Verification items for the finished model (mm, model axes). A direction names the side the tool comes from. Give positions to 0.01 mm unless a question says otherwise; leave off trailing zeros. Loops run counter-clockwise (first coordinate to the right, second up) from the corner with the lowest first, then second, coordinate; pieces in that order, holes last. Notation, with made-up numbers: (-36.75, 0) -> (14.25, 0) arc R16 cw to (14.25, 8) -> close; hole circle Ø10 at (-36.5, 40.5). An arc over 180 degrees is marked (long way). Answer in a Markdown table with one row per item. Add a question column.
Q1. Section check C-C on z = 21.5. Enter the section's corners in (x, y) (3 decimals), and give its area (3 significant figures).
Q2. Gauge pin test, flat ends, axial feed: P1, Ø2, axis at y = -26.5, z = -1.5, coming from the +X side; P2, Ø3, axis at y = -48, z = 18, coming from the -X side; P3, Ø2, axis at x = -3, z = -0.5, coming from the +Y side; P4, Ø12, axis at x = -15, z = 11.5, coming from the +Y side. Record the tip position at first contact, or that the pin passes through.
Q3. Section check D-D on y = -11. Enter the section's corners in (x, z), and give its area (3 significant figures).
Q4. Section check A-A on x = 9.5. Enter the section's corners in (y, z), and give its area (3 significant figures).
Q5. Release check for a two-part mould opening along Y. For faces 4 (the face through (1, -54.61, 13)), 5 (the face through (19.05, -24, -1)), 6 (the face through (51.41, -1.61, 23.87)) record: pulls with the +Y half, pulls with the -Y half, needs draft (parallel to the pull), parting line crosses it, or undercut.
Q6. Material ranges on probe 1 along X at (y, z) = (-9.5, 5.75); probe 2 along X at (y, z) = (-56, 23); probe 3 along Z at (x, y) = (-15.5, -52), recorded low to high.
Q7. Set-up check for faces 1 (the face through (-48, -3.175, 12)), 2 (the face through (-1, -46, 0)), 3 (the face through (0, -41.91, -1)): record each of +Z, -Z, +X, -X, +Y, -Y from which the full face is reachable in a straight line by a thin tool's end or side.
Q8. Section check B-B on y = -4.5. Enter the section's corners in (x, z).
```python
from build123d import *

# Parameters (mm, degrees)
F1_DEPTH  = 25.4
F2_W      = 87.9329293966
F2_H      = 59.3619965534
F3_DEPTH  = 2.54
F4_W      = 8.89
F4_H      = 27.94
F5_DEPTH  = 3.175
F7_DEPTH  = 2.541
F8_R      = 5.08
F9_R      = 2.38125
F10_DEPTH = 3.176


# Not quite as in the source:
# - a feature names something its author has since deleted; it is built from what else it names


with BuildPart() as f1:
    # F0 (on Top) → F1 (new body)
    with BuildSketch(Plane.XY):
        Polygon((38.1, -54.61), (-38.1, -54.61), (-38.1, 0), (-43.9664646983, 0), (-43.9664646983, -59.3619965534), (43.9664646983, -59.3619965534), (43.9664646983, 0), (38.1, 0), align=None)
    extrude(amount=F1_DEPTH)

    # F2 (on face) → F3 (join)
    with BuildSketch(Plane(origin=(0, 0, 0), x_dir=(1, 0, 0), z_dir=(0, 0, -1))):
        with Locations((0, 29.6809982767)):
            Rectangle(F2_W, F2_H)
    extrude(amount=F3_DEPTH)

    # F4 (on face) → F5 (join)
    with BuildSketch(Plane(origin=(0, 0, 0), x_dir=(-1, 0, 0), z_dir=(0, 1, 0))):
        with Locations((-48.4114646983, 11.43)):
            Rectangle(F4_W, F4_H)
        with Locations((48.4114646983, 11.43)):
            Rectangle(F4_W, F4_H)
    extrude(amount=-F5_DEPTH)

    # F6 (on face) → F7 (cut, through all)
    with BuildSketch(Plane.XY):
        Polygon((0, -6.35), (-19.05, -6.35), (-19.05, -41.91), (0, -41.91), (19.05, -41.91), (19.05, -6.35), align=None)
    extrude(amount=-F7_DEPTH, mode=Mode.SUBTRACT)

    # F8
    f8_edges = [f1.edges().sort_by_distance(p)[0] for p in [
        (52.856465, -1.5875, 25.4),
        (-52.856465, -1.5875, 25.4),
        (-52.856465, -1.5875, -2.54),
        (52.856465, -1.5875, -2.54),
    ]]
    fillet(f8_edges, radius=F8_R)

    # F9 (on face) → F10 (cut, through all)
    with BuildSketch(Plane.XZ.offset(3.175)):
        with Locations((48.4114646983, 20.32)):
            Circle(F9_R)
        with Locations((48.4114646983, 2.54)):
            Circle(F9_R)
        with Locations((-48.4114646983, 2.54)):
            Circle(F9_R)
        with Locations((-48.4114646983, 20.32)):
            Circle(F9_R)
    extrude(amount=-F10_DEPTH, mode=Mode.SUBTRACT)


solid = f1.part
```
Taken from the geometry:
| question | item | result |
|---|---|---|
| 1 | outline | (-52.718, -3.175) -> (-50.48, -3.175) -> (-50.48, 0) -> (-52.718, 0) -> close; (-46.343, -3.175) -> (-43.966, -3.175) -> (-43.966, -59.362) -> (43.966, -59.362) -> (43.966, -3.175) -> (46.343, -3.175) -> (46.343, 0) -> (38.1, 0) -> (38.1, -54.61) -> (-38.1, -54.61) -> (-38.1, 0) -> (-46.343, 0) -> close; (50.48, -3.175) -> (52.718, -3.175) -> (52.718, 0) -> (50.48, 0) -> close |
| 1 | area | 1,090 mm² |
| 2 | P1 | stops at x = 43.97 |
| 2 | P2 | stops at x = -43.97 |
| 2 | P3 | stops at y = 0 |
| 2 | P4 | stops at y = -54.61 |
| 3 | outline | (-43.97, -2.54) -> (-19.05, -2.54) -> (-19.05, 0) -> (-38.1, 0) -> (-38.1, 25.4) -> (-43.97, 25.4) -> close; (19.05, -2.54) -> (43.97, -2.54) -> (43.97, 25.4) -> (38.1, 25.4) -> (38.1, 0) -> (19.05, 0) -> close |
| 3 | area | 425 mm² |
| 4 | outline | (-59.36, -2.54) -> (-41.91, -2.54) -> (-41.91, 0) -> (-54.61, 0) -> (-54.61, 25.4) -> (-59.36, 25.4) -> close; (-6.35, -2.54) -> (0, -2.54) -> (0, 0) -> (-6.35, 0) -> close |
| 4 | area | 181 mm² |
| 5 | face 4 | pulls with the +Y half |
| 5 | face 5 | undercut |
| 5 | face 6 | needs draft |
| 6 | probe 1 | x = -43.97 to -38.1, 38.1 to 43.97 |
| 6 | probe 2 | x = -43.97 to 43.97 |
| 6 | probe 3 | z = -2.54 to 0 |
| 7 | face 1 | +Z, -Z, -X, -Y |
| 7 | face 2 | +Z, +Y |
| 7 | face 3 | +Z, -Z |
| 8 | outline | (-43.97, -2.54) -> (43.97, -2.54) -> (43.97, 25.4) -> (38.1, 25.4) -> (38.1, 0) -> (-38.1, 0) -> (-38.1, 25.4) -> (-43.97, 25.4) -> close |
